Check sheet for the modelled part. Datum: model origin and axes. Units: mm. Face numbers are marked on the shaded views. A direction names the side the tool comes from. Round coordinates to 2 decimals unless told otherwise and drop trailing zeros. Write each loop counter-clockwise with the first axis right and the second up, starting at its lowest first coordinate (ties: lowest second). Pieces come first, ordered by that corner, then holes. Notation, with made-up numbers: M 88,45.5 L 132,45.5 A15 cw 132,67.5 Z; hole C 35,35.25 d9. An arc over 180 degrees is marked long. Put each result on its own line as item: value.
```python
from build123d import *

# Parameters (mm, degrees)
EXTRUSION1_DEPTH = 21
ESQUISSE2_W      = 21
ESQUISSE2_H      = 2.5
EXTRUSION2_DEPTH = 7.2
ESQUISSE3_W      = 21
ESQUISSE3_H      = 2.5
EXTRUSION3_DEPTH = 7.2
EXTRUSION4_REACH = 62.641
ESQUISSE4_R      = 2.25
CONG_1_R         = 1
CONG_2_R         = 2
ESQUISSE5_R      = 3
EXTRUSION5_DEPTH = 6
ESQUISSE7_R      = 6.75
EXTRUSION6_DEPTH = 2
CHANFREIN1_SIZE2 = 1.5
CHANFREIN1_SIZE  = 2
EXTRUSION7_REACH = 62.641
ESQUISSE8_W      = 1
ESQUISSE8_H      = 2.5
CONG_3_R         = 0.5
ESQUISSE9_R      = 7
ESQUISSE9_R_2    = 1.5
EXTRUSION8_DEPTH = 2.4
CONG_4_R         = 0.5


with BuildPart() as part:
    # Esquisse1 → Extrusion1 (new body)
    with BuildSketch(Plane.XY):
        Polygon((0, 0), (40.5, 0), (40.5, 34.3), (33, 39.8), (0, 39.8), align=None)
    extrude(amount=-EXTRUSION1_DEPTH)

    # Esquisse2 → Extrusion2 (add)
    with BuildSketch(Plane(origin=(40.5, 0, 0), x_dir=(0, 0, -1), z_dir=(1, 0, 0))):
        with Locations((10.5, 29.75)):
            Rectangle(ESQUISSE2_W, ESQUISSE2_H)
    extrude(amount=EXTRUSION2_DEPTH)

    # Esquisse3 → Extrusion3 (add)
    with BuildSketch(Plane.ZY):
        with Locations((-10.5, 29.75)):
            Rectangle(ESQUISSE3_W, ESQUISSE3_H)
    extrude(amount=EXTRUSION3_DEPTH)

    # Esquisse4 → Extrusion4 (cut, up to next)
    with BuildSketch(Plane(origin=(0, 31, 0), x_dir=(-1, 0, 0), z_dir=(0, 1, 0)), mode=Mode.PRIVATE) as extrusion4_sk1:
        with Locations((4.5, -15.5)):
            Circle(ESQUISSE4_R)
    extrusion4_tool1 = extrude(extrusion4_sk1.sketch, amount=-EXTRUSION4_REACH, mode=Mode.PRIVATE) & part.part
    # Esquisse4 → Extrusion4 (cut, up to next)
    with BuildSketch(Plane(origin=(0, 31, 0), x_dir=(-1, 0, 0), z_dir=(0, 1, 0)), mode=Mode.PRIVATE) as extrusion4_sk2:
        with Locations(Location((-45, -15.5, 0), (0, 0, 90))):
            Circle(ESQUISSE4_R)
    extrusion4_tool2 = extrude(extrusion4_sk2.sketch, amount=-EXTRUSION4_REACH, mode=Mode.PRIVATE) & part.part
    # Esquisse4 → Extrusion4 (cut, up to next)
    with BuildSketch(Plane(origin=(0, 31, 0), x_dir=(-1, 0, 0), z_dir=(0, 1, 0)), mode=Mode.PRIVATE) as extrusion4_sk3:
        with Locations((-45, -5.5)):
            Circle(ESQUISSE4_R)
    extrusion4_tool3 = extrude(extrusion4_sk3.sketch, amount=-EXTRUSION4_REACH, mode=Mode.PRIVATE) & part.part
    # Esquisse4 → Extrusion4 (cut, up to next)
    with BuildSketch(Plane(origin=(0, 31, 0), x_dir=(-1, 0, 0), z_dir=(0, 1, 0)), mode=Mode.PRIVATE) as extrusion4_sk4:
        with Locations(Location((4.5, -5.5, 0), (0, 0, 90))):
            Circle(ESQUISSE4_R)
    extrusion4_tool4 = extrude(extrusion4_sk4.sketch, amount=-EXTRUSION4_REACH, mode=Mode.PRIVATE) & part.part
    add(extrusion4_tool1.solids().sort_by_distance((-4.5, 31, -15.5))[0], mode=Mode.SUBTRACT)
    add(extrusion4_tool2.solids().sort_by_distance((45, 31, -15.5))[0], mode=Mode.SUBTRACT)
    add(extrusion4_tool3.solids().sort_by_distance((45, 31, -5.5))[0], mode=Mode.SUBTRACT)
    add(extrusion4_tool4.solids().sort_by_distance((-4.5, 31, -5.5))[0], mode=Mode.SUBTRACT)

    # Congé1
    cong_1_edges = [part.edges().sort_by_distance(p)[0] for p in [
        (47.7, 29.75, 0),
        (47.7, 29.75, -21),
        (-7.2, 29.75, -21),
        (-7.2, 29.75, 0),
    ]]
    fillet(cong_1_edges, radius=CONG_1_R)

    # Congé2
    cong_2_edges = [part.edges().sort_by_distance(p)[0] for p in [
        (0, 35.4, -21),
        (0, 14.25, -21),
        (0, 35.4, 0),
        (0, 14.25, 0),
        (40.5, 32.65, 0),
        (40.5, 14.25, 0),
        (40.5, 32.65, -21),
        (40.5, 14.25, -21),
    ]]
    fillet(cong_2_edges, radius=CONG_2_R)

    # Esquisse5 → Extrusion5 (add)
    with BuildSketch(Plane(origin=(0, 39.8, 0), x_dir=(-1, 0, 0), z_dir=(0, 1, 0))):
        with Locations((-10.2, -10.5)):
            Circle(ESQUISSE5_R)
    extrude(amount=EXTRUSION5_DEPTH)

    # Esquisse7 → Extrusion6 (add)
    with BuildSketch(Plane(origin=(0, 39.8, 0), x_dir=(-1, 0, 0), z_dir=(0, 1, 0))):
        with Locations((-10.2, -10.5)):
            Circle(ESQUISSE7_R)
    extrude(amount=EXTRUSION6_DEPTH)

    # Chanfrein1
    chanfrein1_edges = [part.edges().sort_by_distance(p)[0] for p in [
        (16.95, 41.8, -10.5),
    ]]
    chanfrein1_side = [part.faces().sort_by_distance(p)[0] for p in [
        (16.95, 41.77, -10.5),
    ]]
    chamfer(chanfrein1_edges, length=CHANFREIN1_SIZE - 0.0001, length2=CHANFREIN1_SIZE2 - 0.0001, reference=chanfrein1_side[0])  # a hair under: the kernel refuses the full size

    # Esquisse8 → Extrusion7 (cut, up to next)
    with BuildSketch(Plane(origin=(0, 31, 0), x_dir=(-1, 0, 0), z_dir=(0, 1, 0)), mode=Mode.PRIVATE) as extrusion7_sk1:
        with Locations((6.7, -15.5)):
            Rectangle(ESQUISSE8_W, ESQUISSE8_H)
    extrusion7_tool1 = extrude(extrusion7_sk1.sketch, amount=-EXTRUSION7_REACH, mode=Mode.PRIVATE) & part.part
    # Esquisse8 → Extrusion7 (cut, up to next)
    with BuildSketch(Plane(origin=(0, 31, 0), x_dir=(-1, 0, 0), z_dir=(0, 1, 0)), mode=Mode.PRIVATE) as extrusion7_sk2:
        with Locations((6.7, -5.5)):
            Rectangle(ESQUISSE8_W, ESQUISSE8_H)
    extrusion7_tool2 = extrude(extrusion7_sk2.sketch, amount=-EXTRUSION7_REACH, mode=Mode.PRIVATE) & part.part
    # Esquisse8 → Extrusion7 (cut, up to next)
    with BuildSketch(Plane(origin=(0, 31, 0), x_dir=(-1, 0, 0), z_dir=(0, 1, 0)), mode=Mode.PRIVATE) as extrusion7_sk3:
        with Locations((-47.2, -15.5)):
            Rectangle(ESQUISSE8_W, ESQUISSE8_H)
    extrusion7_tool3 = extrude(extrusion7_sk3.sketch, amount=-EXTRUSION7_REACH, mode=Mode.PRIVATE) & part.part
    # Esquisse8 → Extrusion7 (cut, up to next)
    with BuildSketch(Plane(origin=(0, 31, 0), x_dir=(-1, 0, 0), z_dir=(0, 1, 0)), mode=Mode.PRIVATE) as extrusion7_sk4:
        with Locations((-47.2, -5.5)):
            Rectangle(ESQUISSE8_W, ESQUISSE8_H)
    extrusion7_tool4 = extrude(extrusion7_sk4.sketch, amount=-EXTRUSION7_REACH, mode=Mode.PRIVATE) & part.part
    add(extrusion7_tool1.solids().sort_by_distance((-6.7, 31, -15.5))[0], mode=Mode.SUBTRACT)
    add(extrusion7_tool2.solids().sort_by_distance((-6.7, 31, -5.5))[0], mode=Mode.SUBTRACT)
    add(extrusion7_tool3.solids().sort_by_distance((47.2, 31, -15.5))[0], mode=Mode.SUBTRACT)
    add(extrusion7_tool4.solids().sort_by_distance((47.2, 31, -5.5))[0], mode=Mode.SUBTRACT)

    # Congé3
    cong_3_edges = [part.edges().sort_by_distance(p)[0] for p in [
        (-7.2, 29.75, -14.25),
        (-7.2, 29.75, -16.75),
        (-6.370828693, 29.75, -16.75),
        (-6.370828693, 29.75, -14.25),
        (-6.370828693, 29.75, -6.75),
        (-6.370828693, 29.75, -4.25),
        (-7.2, 29.75, -6.75),
        (-7.2, 29.75, -4.25),
        (46.870828693, 29.75, -14.25),
        (46.870828693, 29.75, -16.75),
        (47.7, 29.75, -14.25),
        (47.7, 29.75, -16.75),
        (47.7, 29.75, -6.75),
        (47.7, 29.75, -4.25),
        (46.870828693, 29.75, -6.75),
        (46.870828693, 29.75, -4.25),
    ]]
    fillet(cong_3_edges, radius=CONG_3_R)

    # Esquisse9 → Extrusion8 (add)
    with BuildSketch(Plane.XZ):
        with Locations(Location((10.2, -10.5, 0), (0, 0, 270))):
            Circle(ESQUISSE9_R)
        with Locations(Location((10.2, -10.5, 0), (0, 0, 270))):
            Circle(ESQUISSE9_R_2, mode=Mode.SUBTRACT)
    extrude(amount=EXTRUSION8_DEPTH)

    # Congé4
    cong_4_edges = [part.edges().sort_by_distance(p)[0] for p in [
        (10.2, -2.4, -3.5),
    ]]
    fillet(cong_4_edges, radius=CONG_4_R)


solid = part.part
```
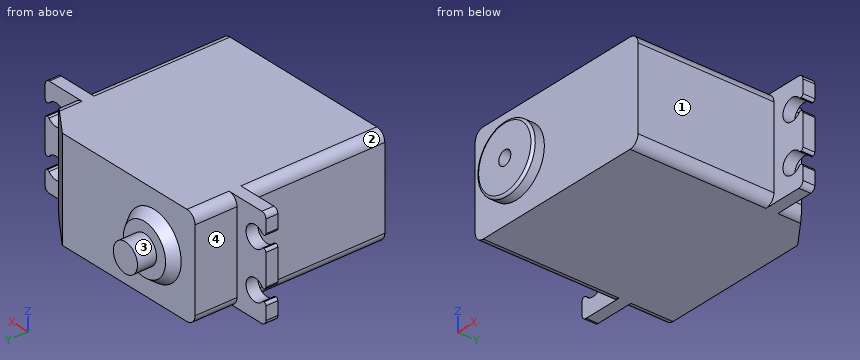
1. Access from +Z, -Z, +X, -X, +Y, -Y to the whole of each face (thin tool, end or side, straight path). Record for the marked faces 1, 2, 3 and 4.
Computed values:
face 1: +Z, -Z, +X, -Y
face 2: +Z, -X, -Y
face 3: +Y
face 4: +Z, -Z, -X, +Y
2. Depth check by flat-ended pin: pin 1 Ø12 at (y, z) = (13.5, -17) entering from +X; pin 2 Ø2 at (x, z) = (22, -11.5) entering from -Y; pin 3 Ø1 at (x, y) = (-1.5, 14.5) entering from -Z; pin 4 Ø3 at (x, z) = (45, -13) entering from +Y. Enter the tip coordinate at first touch or a pass-through.
Computed values:
pin 1: stops at x = 40.5
pin 2: stops at y = 0
pin 3: passes through
pin 4: stops at y = 31
3. Cross-section at A-A (x = 45). Enter the section's corners in (y, z), then the cut area to 3 significant figures.
Computed values:
outline: M 28.5,-21 L 31,-21 L 31,-17.75 L 28.5,-17.75 Z; M 28.5,-13.25 L 31,-13.25 L 31,-7.75 L 28.5,-7.75 Z; M 28.5,-3.25 L 31,-3.25 L 31,0 L 28.5,0 Z
area: 30.0 mm2
4. Cross-section at B-B (y = 22). Enter the section's corners in (x, z), then the cut area to 3 significant figures.
Computed values:
outline: M 0,-19 A2 ccw 2,-21 L 38.5,-21 A2 ccw 40.5,-19 L 40.5,-2 A2 ccw 38.5,0 L 2,0 A2 ccw 0,-2 Z
area: 847 mm2
5. Scan lines: probe 1 along Z at (x, y) = (-4.5, 30.2); probe 2 along Y at (x, z) = (6, -11.5); probe 3 along X at (y, z) = (29.4, -15.5). Record each from-to range of solid material in increasing order.
Computed values:
probe 1: z = -21 to -17.75, -13.25 to -7.75, -3.25 to 0
probe 2: y = -2.4 to 41.8
probe 3: x = -2.25 to 42.75
